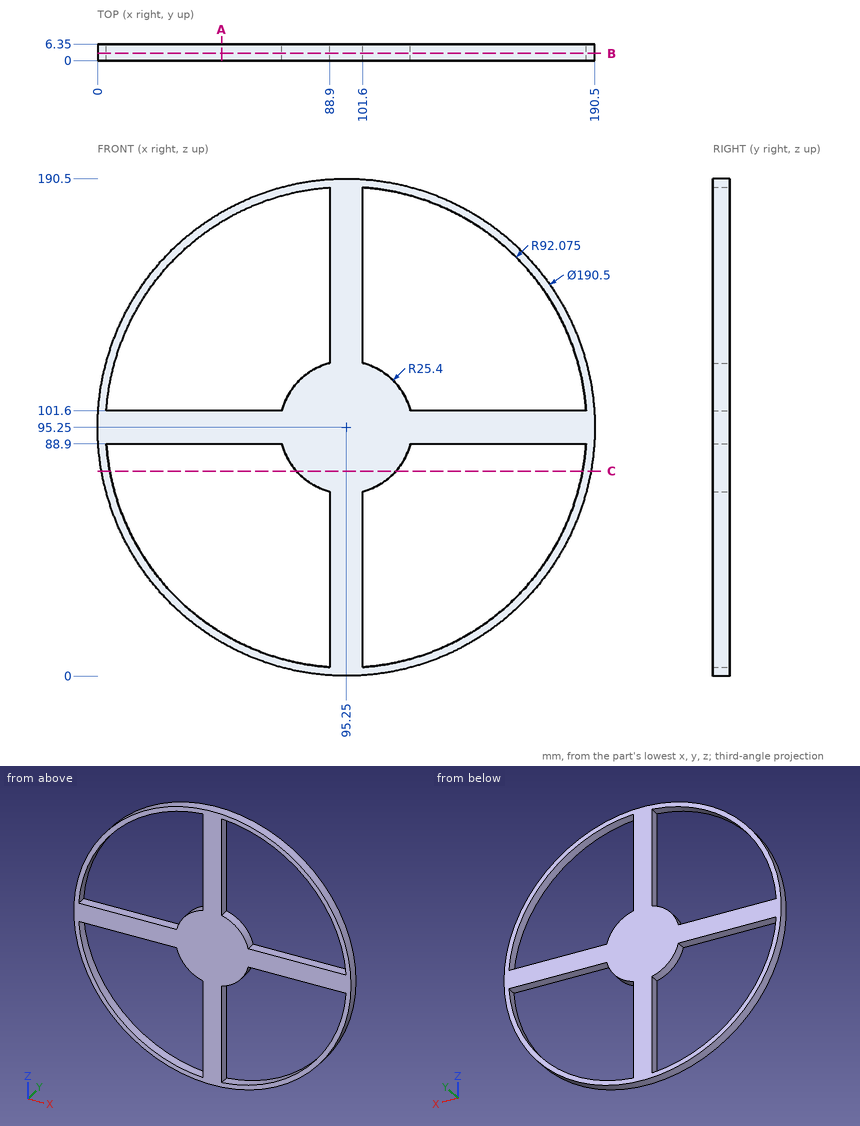
Could you check a few things on this drawing? It's one solid part, dimensions in mm from its lowest x, y, z. Round coordinates to 2 decimals unless told otherwise and drop trailing zeros. Order: outer loops, then holes, each group sorted by start corner. A loop starts at its lowest first (then second) coordinate and runs counter-clockwise, first axis right, second up.
Q1. I'm going to push flat-ended pins straight in: P1, Ø1.9, axis at y = 4, z = 42, coming from the -X side; P2, Ø1, axis at x = 107, y = 1, coming from the +Z side; P3, Ø3, axis at y = 2, z = 20, coming from the -X side. Where does each tip first touch, or does it pass through?
Geometry says:
P1: stops at x = 15.64
P2: stops at z = 189.83
P3: stops at x = 34.97
Q2. Please list where these lines run through material, in increasing order: probe 1 along Z at (x, y) = (140, 0.5); probe 2 along Z at (x, y) = (23, 0.75); probe 3 along X at (y, z) = (1.5, 51).
Geometry says:
probe 1: z = 11.17 to 14.78, 88.9 to 101.6, 175.72 to 179.33
probe 2: z = 33.18 to 38.17, 88.9 to 101.6, 152.33 to 157.32
probe 3: x = 10.9 to 14.51, 88.9 to 101.6, 175.99 to 179.6
Q3. Imagine slicing it at A-A, the plane x = 47.5. List the corners of the cut face in (y, z) for me.
Geometry says:
outline: (0, 12.83) - (6.35, 12.83) - (6.35, 16.52) - (0, 16.52) - close; (0, 88.9) - (6.35, 88.9) - (6.35, 101.6) - (0, 101.6) - close; (0, 173.98) - (6.35, 173.98) - (6.35, 177.67) - (0, 177.67) - close
Q4. Imagine slicing it at B-B, the plane y = 2.75. List the corners of the cut face in (x, z) for me (3 decimals).
Geometry says:
outline: circle Ø190.5 at (95.25, 95.25); hole (3.394, 88.9) arc R92.075 ccw to (88.9, 3.394) - (88.9, 70.657) arc R25.4 cw to (70.657, 88.9) - close; hole (3.394, 101.6) - (70.657, 101.6) arc R25.4 cw to (88.9, 119.843) - (88.9, 187.106) arc R92.075 ccw to start; hole (101.6, 3.394) arc R92.075 ccw to (187.106, 88.9) - (119.843, 88.9) arc R25.4 cw to (101.6, 70.657) - close; hole (101.6, 119.843) arc R25.4 cw to (119.843, 101.6) - (187.106, 101.6) arc R92.075 ccw to (101.6, 187.106) - close
Q5. Imagine slicing it at C-C, the plane z = 78.5. List the corners of the cut face in (x, y) for me, then the cut area to 3 significant figures.
Geometry says:
outline: (1.48, 0) - (4.71, 0) - (4.71, 6.35) - (1.48, 6.35) - close; (76.16, 0) - (114.34, 0) - (114.34, 6.35) - (76.16, 6.35) - close; (185.79, 0) - (189.02, 0) - (189.02, 6.35) - (185.79, 6.35) - close
area: 283 mm2
